Work out the finished part from the listing and answer in its coordinate system (mm). A direction names the side the tool comes from. Round coordinates to 2 decimals unless told otherwise and drop trailing zeros. Write each loop counter-clockwise with the first axis right and the second up, starting at its lowest first coordinate (ties: lowest second). Pieces come first, ordered by that corner, then holes. Notation, with made-up numbers: (-24, 51.5) -> (9, 51.5) arc R33 cw to (9, 84.5) -> close; hole circle Ø5 at (27.5, 37.5). An arc over 180 degrees is marked (long way). One line per question, with ' | ' between items. Start each with the question number.
```python
from build123d import *

# Parameters (mm, degrees)
CROQUIS1_W              = 25
CROQUIS1_H              = 30
SALIENTE_EXTRUIR1_DEPTH = 3
CROQUIS2_R              = 1.05
SALIENTE_EXTRUIR2_DEPTH = 3
SALIENTE_EXTRUIR3_DEPTH = 2
CROQUIS4_R              = 1.5
SALIENTE_EXTRUIR4_DEPTH = 4
CROQUIS5_R              = 1.1
SALIENTE_EXTRUIR5_DEPTH = 3


with BuildPart() as part:
    # Croquis1 → Saliente-Extruir1 (new body)
    with BuildSketch(Plane.XY):
        Rectangle(CROQUIS1_W, CROQUIS1_H)
    extrude(amount=SALIENTE_EXTRUIR1_DEPTH)

    # Croquis2 → Saliente-Extruir2 (add)
    with BuildSketch(Plane.XY.offset(3)):
        with Locations(Location((-7.5, 0, 0), (0, 0, 180))):
            Circle(CROQUIS2_R)
        with Locations(Location((-2.5, 0, 0), (0, 0, 180))):
            Circle(CROQUIS2_R)
        with Locations(Location((2.5, 0, 0), (0, 0, 180))):
            Circle(CROQUIS2_R)
        with Locations(Location((7.5, 0, 0), (0, 0, 180))):
            Circle(CROQUIS2_R)
    extrude(amount=SALIENTE_EXTRUIR2_DEPTH)

    # Croquis3 → Saliente-Extruir3 (add)
    with BuildSketch(Plane(origin=(12.5, 0, 0), x_dir=(0, 0, -1), z_dir=(1, 0, 0))):
        with BuildLine():
            Line((-3, 3), (-3, 2.5))
            ThreePointArc((-3, 2.5), (-0.5, 0), (-3, -2.5))
            Line((-3, -2.5), (-3, -3))
            ThreePointArc((-3, -3), (0, 0), (-3, 3))
        make_face()
    extrude(amount=SALIENTE_EXTRUIR3_DEPTH)

    # Croquis4 → Saliente-Extruir4 (add)
    with BuildSketch(Plane(origin=(0, 0, 0), x_dir=(-1, 0, 0), z_dir=(0, 0, -1))):
        with Locations((10.5, 13)):
            Circle(CROQUIS4_R)
        with Locations((-10.5, 13)):
            Circle(CROQUIS4_R)
        with Locations((-10.5, 0.5)):
            Circle(CROQUIS4_R)
        with Locations((10.5, 0.5)):
            Circle(CROQUIS4_R)
    extrude(amount=SALIENTE_EXTRUIR4_DEPTH)

    # Croquis5 → Saliente-Extruir5 (add)
    with BuildSketch(Plane(origin=(0, 0, -4), x_dir=(-1, 0, 0), z_dir=(0, 0, -1))):
        with Locations((10.5, 13)):
            Circle(CROQUIS5_R)
        with Locations((-10.5, 13)):
            Circle(CROQUIS5_R)
        with Locations((-10.5, 0.5)):
            Circle(CROQUIS5_R)
        with Locations((10.5, 0.5)):
            Circle(CROQUIS5_R)
    extrude(amount=SALIENTE_EXTRUIR5_DEPTH)


solid = part.part
```
(1) A cutting plane is placed at C-C, the plane y = 13. Determine the outline of the cut face in (x, z), then the cut area to 3 significant figures.
(2) For faces 1 (the cylindrical face through (13.5, 0.1, 0.5)), 2 (the cylindrical face through (-9, 0.57, -1.97)), 3 (the cylindrical face through (-3.5, -0.32, 4.48)), determine the directions among +Z, -Z, +X, -X, +Y, -Y from which every point of the face is accessible in a straight line to the end or side of a thin tool.
(3) A cutting plane is placed at B-B, the plane z = -6. Determine the outline of the cut face in (x, y).
(4) A cutting plane is placed at D-D, the plane z = 1.75. Determine the outline of the cut face in (x, y).
(5) Given pin 1 Ø5 at (x, y) = (10.5, -11.5) entering from +Z; pin 2 Ø13.5 at (x, y) = (2.5, 4) entering from +Z; pin 3 Ø4 at (x, y) = (7.5, -7.5) entering from -Z; pin 4 Ø2.5 at (y, z) = (10, 1.5) entering from +X, each flat-ended and moving along its own axis, determine where each tip first touches the part or whether it passes through.
(6) A cutting plane is placed at A-A, the plane x = 10.5. Determine the outline of the cut face in (y, z), then the cut area to 3 significant figures.
(7) The mould has two halves that part along Y. Classify faces 4 (the cylindrical face through (-11.516, 0.079, -5.479)), 5 (the cylindrical face through (-6.45, -0.05, 4.48)), 6 (the flat face through (-10, 1, -7)): +Y half, -Y half, draft (parallel to the pull), parting line (faces both ways), or undercut.
(8) Consider L1, parallel to X at y = -0.75, z = 3.5; L2, parallel to Z at x = -1.75, y = -4.75; L3, parallel to Y at x = -10.75, z = -1.75. Determine where each line is inside the solid, lowest interval first.
Returned:
1) outline: (-12.5, 0) -> (-12, 0) -> (-12, -4) -> (-11.6, -4) -> (-11.6, -7) -> (-9.4, -7) -> (-9.4, -4) -> (-9, -4) -> (-9, 0) -> (9, 0) -> (9, -4) -> (9.4, -4) -> (9.4, -7) -> (11.6, -7) -> (11.6, -4) -> (12, -4) -> (12, 0) -> (12.5, 0) -> (12.5, 3) -> (-12.5, 3) -> close | area: 112 mm2
2) face 1: +Z, +X | face 2: -Z | face 3: +Z
3) outline: circle Ø2.2 at (-10.5, 0.5); circle Ø2.2 at (-10.5, 13); circle Ø2.2 at (10.5, 0.5); circle Ø2.2 at (10.5, 13)
4) outline: (-12.5, -15) -> (12.5, -15) -> (12.5, -2.73) -> (14.5, -2.73) -> (14.5, -2.17) -> (12.5, -2.17) -> (12.5, 2.17) -> (14.5, 2.17) -> (14.5, 2.73) -> (12.5, 2.73) -> (12.5, 15) -> (-12.5, 15) -> close
5) pin 1: z = 3 | pin 2: z = 6 | pin 3: z = 0 | pin 4: x = 12.5
6) outline: (-15, 0) -> (-1, 0) -> (-1, -4) -> (-0.6, -4) -> (-0.6, -7) -> (1.6, -7) -> (1.6, -4) -> (2, -4) -> (2, 0) -> (11.5, 0) -> (11.5, -4) -> (11.9, -4) -> (11.9, -7) -> (14.1, -7) -> (14.1, -4) -> (14.5, -4) -> (14.5, 0) -> (15, 0) -> (15, 3) -> (-15, 3) -> close | area: 127 mm2
7) face 4: undercut | face 5: parting line | face 6: draft
8) L1: -8.23 to -6.77, -3.23 to -1.77, 1.77 to 3.23, 6.77 to 8.23 | L2: 0 to 3 | L3: -0.98 to 1.98, 11.52 to 14.48
